Input: part model. Units: mm. Frame: model coordinates. A direction names the side the tool comes from. Coordinates: 2 decimals unless noted, no trailing zeros. Order: outer loops, then holes, each group sorted by start corner. A loop starts at its lowest first (then second) coordinate and runs counter-clockwise, first axis right, second up. Notation, with made-up numbers: (75, 1) - (105, 1) arc R5 cw to (105, 5) - close; hole circle Ø9 at (32, 25.25). An arc over 180 degrees is marked (long way). Answer as CSV lines item,"result". Start each with the question number.
Item 1: Section D-D (y = 11.25). Output: boundary loops of the cut face in (x, z).
Item 2: Access query for faces 1 (the flat face through (3, 8, -13)), 2 (the flat face through (0, 4.101, 0)), 3 (the flat face through (-10, 6, -15)), 4 (the flat face through (-10, 6, 15)). Directions: +Z, -Z, +X, -X, +Y, -Y. A direction counts if a zero-diameter tool reaches every point of the face in a straight line with its end or side. Return the directions, or none.
Item 3: First-contact query: pin 1 (3 mm diameter, centred on x = -8, y = 5, fed in from +Z); pin 2 (6.5 mm diameter, centred on x = -0.5, y = 8.5, fed in from -Z); pin 3 (2.5 mm diameter, centred on x = -2, z = 7.5, fed in from -Y). Flat tips, straight axial feed; report the tip coordinate or a pass-through.
Item 4: Section A-A (y = 18.5). Output: boundary loops of the cut face in (x, z).
Item 5: Draft query along Z for faces 5 (the cylindrical face through (-10.426, 6.439, -8.496)), 6 (the flat face through (9, 6, -15)), 7 (the flat face through (6, 2.1, 0.2)), 8 (the cylindrical face through (-10.476, 6.439, 8.632)). Return one class per face: +Z half, -Z half, draft (parallel to the pull), parting line (faces both ways), or undercut.
Item 6: Section B-B (x = -12). Output: boundary loops of the cut face in (y, z).
Item 7: Section C-C (z = -8). Output: boundary loops of the cut face in (x, y), and give its area (3 significant figures).
Item 8: Material intervals for line 1 along Z through (x, y) = (-12, 9.5); line 2 along Z through (x, y) = (-13, 5); line 3 along X through (y, z) = (9.5, 12), sorted ascending.
from build123d import *

# Parameters (mm, degrees)
BOSS_EXTRUDE1_DEPTH = 15
SKETCH2_R           = 1.65
CUT_EXTRUDE1_DEPTH  = 12.7
SKETCH3_W           = 4.5
SKETCH3_H           = 7.5
BOSS_EXTRUDE3_DEPTH = 12.7
SKETCH3_7_W         = 6
SKETCH3_7_H         = 3.5
CUT_EXTRUDE4_DEPTH  = 12.7


with BuildPart() as part:
    # Sketch1 → Boss-Extrude1 (new body, symmetric)
    with BuildSketch(Plane.XY):
        Polygon((-4, 4.101219331), (4, 4.101219331), (8.101219331, 0), (16, 0), (16, 12.7), (-16, 12.7), (-16, 0), (-8.101219331, 0), align=None)
    extrude(amount=BOSS_EXTRUDE1_DEPTH, both=True)

    # Sketch2 → Cut-Extrude1 (cut)
    with BuildSketch(Plane(origin=(0, 12.7, 0), x_dir=(1, 0, 0), z_dir=(0, 1, 0))):
        with Locations((12, 8)):
            Circle(SKETCH2_R)
        with Locations((12, -8)):
            Circle(SKETCH2_R)
        with Locations((-12, -8)):
            Circle(SKETCH2_R)
        with Locations((-12, 8)):
            Circle(SKETCH2_R)
    extrude(amount=-CUT_EXTRUDE1_DEPTH, mode=Mode.SUBTRACT)

    # Sketch3 → Boss-Extrude3 (add)
    with BuildSketch(Plane(origin=(0, 12.7, 0), x_dir=(1, 0, 0), z_dir=(0, 1, 0))):
        with Locations((5.25, 18.75)):
            Rectangle(SKETCH3_W, SKETCH3_H)
        Polygon((3, -15), (7.5, -15), (7.5, 15), (3, 15), (3, 11.5), (-3, 11.5), (-3, 15), (-7.5, 15), (-7.5, -15), (-3, -15), (-3, -11.5), (3, -11.5), align=None)
        with Locations((-5.25, 18.75)):
            Rectangle(SKETCH3_W, SKETCH3_H)
        with BuildLine():
            Line((2.561737691, 15), (3, 15))
            Line((3, 15), (3, 22.5))
            Line((3, 22.5), (-3, 22.5))
            Line((-3, 22.5), (-3, 15))
            Line((-3, 15), (-2.561737691, 15))
            ThreePointArc((-2.561737691, 15), (-0.508783524, 18.702524621), (2.75, 16))
            ThreePointArc((2.75, 16), (2.702524621, 15.491216476), (2.561737691, 15))
        make_face()
        with BuildLine():
            Line((3, 11.5), (3, 15))
            Line((3, 15), (2.561737691, 15))
            ThreePointArc((2.561737691, 15), (0, 13.25), (-2.561737691, 15))
            Line((-2.561737691, 15), (-3, 15))
            Line((-3, 15), (-3, 11.5))
            Line((-3, 11.5), (3, 11.5))
        make_face()
        with BuildLine():
            Line((-3, -22.5), (3, -22.5))
            Line((3, -22.5), (3, -15))
            Line((3, -15), (2.561737691, -15))
            ThreePointArc((2.561737691, -15), (2.702524621, -15.491216476), (2.75, -16))
            ThreePointArc((2.75, -16), (-0.508783524, -18.702524621), (-2.561737691, -15))
            Line((-2.561737691, -15), (-3, -15))
            Line((-3, -15), (-3, -22.5))
        make_face()
        with Locations((5.25, -18.75)):
            Rectangle(SKETCH3_W, SKETCH3_H)
        with Locations((-5.25, -18.75)):
            Rectangle(SKETCH3_W, SKETCH3_H)
        with BuildLine():
            Line((2.561737691, -15), (3, -15))
            Line((3, -15), (3, -11.5))
            Line((3, -11.5), (-3, -11.5))
            Line((-3, -11.5), (-3, -15))
            Line((-3, -15), (-2.561737691, -15))
            ThreePointArc((-2.561737691, -15), (0, -13.25), (2.561737691, -15))
        make_face()
    extrude(amount=BOSS_EXTRUDE3_DEPTH)

    # Sketch3<7> → Cut-Extrude4 (cut)
    with BuildSketch(Plane(origin=(0, 12.7, 0), x_dir=(1, 0, 0), z_dir=(0, 1, 0))):
        with Locations((0, -13.25)):
            Rectangle(SKETCH3_7_W, SKETCH3_7_H)
        with Locations((0, 13.25)):
            Rectangle(SKETCH3_7_W, SKETCH3_7_H)
    extrude(amount=-CUT_EXTRUDE4_DEPTH, mode=Mode.SUBTRACT)


solid = part.part
Determined:
1,outline,"(-16, -15) - (-3, -15) - (-3, -11.5) - (3, -11.5) - (3, -15) - (16, -15) - (16, 15) - (3, 15) - (3, 11.5) - (-3, 11.5) - (-3, 15) - (-16, 15) - close; hole circle Ø3.3 at (-12, -8); hole circle Ø3.3 at (-12, 8); hole circle Ø3.3 at (12, -8); hole circle Ø3.3 at (12, 8)"
2,face 1,"-Z, -Y"
2,face 2,"+Z, -Z, -Y"
2,face 3,"-Z, +X, -X, -Y"
2,face 4,"+Z, +X, -X, -Y"
3,pin 1,"stops at z = 15"
3,pin 2,"stops at z = -15"
3,pin 3,"stops at y = 4.1"
4,outline,"(-7.5, -22.5) - (7.5, -22.5) - (7.5, 22.5) - (-7.5, 22.5) - close; hole circle Ø5.5 at (0, -16); hole circle Ø5.5 at (0, 16)"
5,face 5,"undercut"
5,face 6,"-Z half"
5,face 7,"draft"
5,face 8,"undercut"
6,outline,"(0, -15) - (12.7, -15) - (12.7, -9.65) - (0, -9.65) - close; (0, -6.35) - (12.7, -6.35) - (12.7, 6.35) - (0, 6.35) - close; (0, 9.65) - (12.7, 9.65) - (12.7, 15) - (0, 15) - close"
7,outline,"(-16, 0) - (-13.65, 0) - (-13.65, 12.7) - (-16, 12.7) - close; (-10.35, 0) - (-8.1, 0) - (-4, 4.1) - (4, 4.1) - (8.1, 0) - (10.35, 0) - (10.35, 12.7) - (7.5, 12.7) - (7.5, 25.4) - (-7.5, 25.4) - (-7.5, 12.7) - (-10.35, 12.7) - close; (13.65, 0) - (16, 0) - (16, 12.7) - (13.65, 12.7) - close"
7,area,"463 mm^2"
8,line 1,"z = -15 to -9.65, -6.35 to 6.35, 9.65 to 15"
8,line 2,"z = -15 to -9.31, -6.69 to 6.69, 9.31 to 15"
8,line 3,"x = -16 to -3, 3 to 16"
